Autodesk Fusion 360 part; units mm, degrees
sketch "Sketch1" plane through (0, 0, 0) normal (0, 0, 1) x (1, 0, 0)
  line L0 (50, 50) -> (-50, 50)
  line L1 (-50, 50) -> (-50, -50)
  line L2 (-50, -50) -> (50, -50)
  line L3 (50, -50) -> (50, 50)
  line L4 (50, 50) -> (-50, -50) construction
  line L5 (-50, 50) -> (50, -50) construction
  line L6 (44.75, 44.75) -> (-44.75, 44.75)
  line L7 (-44.75, 44.75) -> (-44.75, -44.75)
  line L8 (-44.75, -44.75) -> (44.75, -44.75)
  line L9 (44.75, -44.75) -> (44.75, 44.75)
  line L10 (44.75, 44.75) -> (-44.75, -44.75) construction
  line L11 (-44.75, 44.75) -> (44.75, -44.75) construction
  dimension "d1" = 89.5
  dimension "d12" = 89.5
extrude "Extrude1" add sketch "Sketch1" along normal blind 5
extrude "Extrude2" add sketch "Sketch1" along normal blind 8 contours L6 L7 L8 L9
sketch "Sketch2" plane through (0, -50, 0) normal (0, -1, 0) x (1, 0, 0)
  line L0 (-50, 0) -> (50, 0)
  line L1 (50, 0) -> (50, 5)
  line L2 (50, 5) -> (-50, 5)
  line L3 (-50, 5) -> (-50, 0)
  line L4 (1.5, 8) -> (-1.5, 8)
  line L5 (-1.5, 8) -> (-1.5, 2)
  line L6 (-1.5, 2) -> (1.5, 2)
  line L7 (1.5, 2) -> (1.5, 8)
  line L8 (1.5, 8) -> (-1.5, 2) construction
  line L9 (-1.5, 8) -> (1.5, 2) construction
  point P0 (0, 5)
  dimension "d6" = 6
  dimension "d7" = 3
extrude "Extrude3" cut sketch "Sketch2" against normal blind 8 contours L2 L4 L5 L7 | L2 L5 L6 L7
chamfer "Chamfer1" distance 0.5 angle 45 4 edges at (-23.125, -44.75, 8) (-44.75, 0, 8) (23.125, -44.75, 8) (44.75, 0, 8)
chamfer "Chamfer1" distance 0.5 angle 45 1 edges at (0, 44.75, 8)
sketch "Sketch3" plane through (0, 0, 8) normal (0, 0, 1) x (-1, 0, 0)
  line L0 (44.25, 44.25) -> (1.5, 44.25)
  line L1 (1.5, 44.25) -> (1.5, 42)
  line L2 (1.5, 42) -> (-1.5, 42)
  line L3 (-1.5, 42) -> (-1.5, 44.25)
  line L4 (-1.5, 44.25) -> (-44.25, 44.25)
  line L5 (-44.25, 44.25) -> (-44.25, -44.25)
  line L6 (-44.25, -44.25) -> (44.25, -44.25)
  line L7 (44.25, -44.25) -> (44.25, 44.25)
  line L8 (-37.5, -37.5) -> (37.5, -37.5)
  line L9 (37.5, -37.5) -> (37.5, 37.5)
  line L10 (37.5, 37.5) -> (-37.5, 37.5)
  line L11 (-37.5, 37.5) -> (-37.5, -37.5)
  line L12 (-37.5, -37.5) -> (37.5, 37.5) construction
  line L13 (37.5, -37.5) -> (-37.5, 37.5) construction
  dimension "d13" = 75
  dimension "d14" = 75
extrude "Extrude4" cut sketch "Sketch3" against normal blind 4 contours L8 L9 L10 L11
Input: part model. Units: mm. Frame: model coordinates. A direction names the side the tool comes from. Coordinates: 2 decimals unless noted, no trailing zeros. Loops run counter-clockwise (first coordinate to the right, second up) from the corner with the lowest first, then second, coordinate; pieces in that order, holes last. Notation, with made-up numbers: (-11, -34.5) - (36, -34.5) arc R26 ccw to (36, -7.5) - close; hole circle Ø10 at (-30, -16.75). An arc over 180 degrees is marked (long way). Answer in a Markdown table with one row per item. Add a question column.
Item 1: Section query A-A on y = 39.5. Return the cut outline in (x, z).
Item 2: Mould query, pull axis X, two halves, no side actions, for faces 1 (the flat face through (37.5, -1, 6)), 2 (the flat face through (-50, 1, 2)), 3 (the flat face through (-23, -44.75, 6)). Classes: released by +X, released by -X, zero draft, split by the parting line, or undercut.
Item 3: Line query: line 1 along Y through (x, z) = (33.5, 4.75); line 2 along X through (y, z) = (-20.5, 6). Output: solid intervals per line, ascending. Write a range as [from, to].
Item 4: Section query B-B on x = 29.5. Return the cut outline in (y, z).
Item 5: Access query for faces 4 (the flat face through (0, -42, 5)), 5 (the flat face through (-44.75, 1, 6)), 6 (the flat face through (44.75, -1, 6)), 7 (the flat face through (1, 37.5, 6)), 8 (the flat face through (1, 44.75, 6)). Directions: +Z, -Z, +X, -X, +Y, -Y. A direction counts if a zero-diameter tool reaches every point of the face in a straight line with its end or side. Return the directions, or none.
Item 6: Contact query for flat-ended pins moving along their axis: P1, Ø1, axis at x = 12, y = 12, coming from the +Z side; P2, Ø6, axis at x = -19.5, y = 17.5, coming from the -Z side; P3, Ø0.8, axis at y = 7.5, z = 6, coming from the -X side; P4, Ø2, axis at x = 17.5, z = 6.5, coming from the -Y side. Output: stop coordinate, or through.
Recorded:
| question | item | result |
|---|---|---|
| 1 | outline | (-50, 0) - (50, 0) - (50, 5) - (44.75, 5) - (44.75, 7.5) - (44.25, 8) - (-44.25, 8) - (-44.75, 7.5) - (-44.75, 5) - (-50, 5) - close |
| 2 | face 1 | undercut |
| 2 | face 2 | released by -X |
| 2 | face 3 | zero draft |
| 3 | line 1 | [-50, -37.5], [37.5, 50] |
| 3 | line 2 | [-44.75, -37.5], [37.5, 44.75] |
| 4 | outline | (-50, 0) - (50, 0) - (50, 5) - (44.75, 5) - (44.75, 7.5) - (44.25, 8) - (37.5, 8) - (37.5, 4) - (-37.5, 4) - (-37.5, 8) - (-44.25, 8) - (-44.75, 7.5) - (-44.75, 5) - (-50, 5) - close |
| 5 | face 4 | +Z, -Y |
| 5 | face 5 | +Z, -X, +Y, -Y |
| 5 | face 6 | +Z, +X, +Y, -Y |
| 5 | face 7 | +Z |
| 5 | face 8 | +Z, +X, -X, +Y |
| 6 | P1 | z = 4 |
| 6 | P2 | z = 0 |
| 6 | P3 | x = -44.75 |
| 6 | P4 | y = -44.75 |
